```python
from build123d import *

# Parameters (mm, degrees)
F1_DEPTH = 8
F2_R     = 1.5
F3_DEPTH = 25
F5_DEPTH = 3


with BuildPart() as f1:
    # F0 (on Top) → F1 (new body)
    with BuildSketch(Plane.XY):
        with BuildLine():
            ThreePointArc((-1.3455948979, -5), (-2.7842223612, -3.1118759439), (-4.5798539423, -1.5593397432))
            ThreePointArc((-4.5798539423, -1.5593397432), (-12.5002387345, 0.4336426528), (-19.7463435047, -3.3344390538))
            ThreePointArc((-19.7463435047, -3.3344390538), (-18.6438704622, -3.0655634038), (-18, -4))
            ThreePointArc((-18, -4), (-18.2928932188, -4.7071067812), (-19, -5))
            Line((-19, -5), (-1.3455948979, -5))
        make_face()
        with BuildLine():
            ThreePointArc((-18, -4), (-18.6438704622, -3.0655634038), (-19.7463435047, -3.3344390538))
            ThreePointArc((-19.7463435047, -3.3344390538), (-19.9344365962, -3.6438704622), (-20, -4))
            ThreePointArc((-20, -4), (-19.7071067812, -4.7071067812), (-19, -5))
            ThreePointArc((-19, -5), (-18.2928932188, -4.7071067812), (-18, -4))
        make_face()
        with BuildLine():
            ThreePointArc((1.3455948979, -5), (2.7842223453, -3.1118759608), (4.5798539043, -1.5593397698))
            ThreePointArc((4.5798539043, -1.5593397698), (-2.32e-08, -3), (-4.5798539423, -1.5593397432))
            ThreePointArc((-4.5798539423, -1.5593397432), (-2.7842223612, -3.1118759439), (-1.3455948979, -5))
            Line((-1.3455948979, -5), (1.3455948979, -5))
        make_face()
        with BuildLine():
            ThreePointArc((19.7463434531, -3.3344389961), (12.5002386731, 0.43364266), (4.5798539043, -1.5593397698))
            ThreePointArc((4.5798539043, -1.5593397698), (2.7842223453, -3.1118759608), (1.3455948979, -5))
            Line((1.3455948979, -5), (19, -5))
            ThreePointArc((19, -5), (18.0874319193, -3.5910751927), (19.7463434531, -3.3344389961))
        make_face()
        with BuildLine():
            ThreePointArc((19, -5), (19.7071067812, -4.7071067812), (20, -4))
            ThreePointArc((20, -4), (19.9344365824, -3.6438704261), (19.7463434531, -3.3344389961))
            ThreePointArc((19.7463434531, -3.3344389961), (18.0874319193, -3.5910751927), (19, -5))
        make_face()
    extrude(amount=F1_DEPTH)

    # F2 (on face) → F3 (cut)
    with BuildSketch(Plane.XZ.offset(5)):
        with Locations((-15, 4)):
            Circle(F2_R)
        with Locations((15, 4)):
            Circle(F2_R)
    extrude(amount=-F3_DEPTH, mode=Mode.SUBTRACT)

    # F4 (on face) → F5 (cut)
    with BuildSketch(Plane.XZ.offset(5)):
        Polygon((-12.25, 2.4122867597), (-12.25, 5.5877132403), (-15, 7.1754264805), (-17.75, 5.5877132403), (-17.75, 2.4122867597), (-15, 0.8245735195), align=None)
        Polygon((12.25, 5.5877132403), (12.25, 2.4122867597), (15, 0.8245735195), (17.75, 2.4122867597), (17.75, 5.5877132403), (15, 7.1754264805), align=None)
    extrude(amount=-F5_DEPTH, mode=Mode.SUBTRACT)


solid = f1.part
```
Geometry: final body of the model. Coordinates: model frame, mm. A direction names the side the tool comes from. Round coordinates to 2 decimals unless told otherwise and drop trailing zeros. Loops run counter-clockwise (first coordinate to the right, second up) from the corner with the lowest first, then second, coordinate; pieces in that order, holes last.
Item 1: Section C-C, the plane z = 4. Output: boundary loops of the cut face in (x, y).
Checked values:
outline: (-19.75, -3.33) arc R1 ccw to (-19, -5) - (-17.75, -5) - (-17.75, -2) - (-16.5, -2) - (-16.5, -0.8) arc R11.5 ccw to start; (-13.5, -2) - (-12.25, -2) - (-12.25, -5) - (12.25, -5) - (12.25, -2) - (13.5, -2) - (13.5, 0.27) arc R11.5 ccw to (4.58, -1.56) arc R8 cw to (-4.58, -1.56) arc R11.5 ccw to (-13.5, 0.27) - close; (16.5, -2) - (17.75, -2) - (17.75, -5) - (19, -5) arc R1 ccw to (19.75, -3.33) arc R11.5 ccw to (16.5, -0.8) - close
Item 2: Section D-D, the plane z = 2. Output: boundary loops of the cut face in (x, y).
Checked values:
outline: (-19.75, -3.33) arc R1 ccw to (-19, -5) - (-17.04, -5) - (-17.04, -2) - (-12.96, -2) - (-12.96, -5) - (12.96, -5) - (12.96, -2) - (17.04, -2) - (17.04, -5) - (19, -5) arc R1 ccw to (19.75, -3.33) arc R11.5 ccw to (4.58, -1.56) arc R8 cw to (-4.58, -1.56) arc R11.5 ccw to start
Item 3: Section A-A, the plane y = -4.6. Output: boundary loops of the cut face in (x, z).
Checked values:
outline: (-19.8, 0) - (19.8, 0) - (19.8, 8) - (-19.8, 8) - close; hole (-17.75, 2.41) - (-15, 0.82) - (-12.25, 2.41) - (-12.25, 5.59) - (-15, 7.18) - (-17.75, 5.59) - close; hole (12.25, 2.41) - (15, 0.82) - (17.75, 2.41) - (17.75, 5.59) - (15, 7.18) - (12.25, 5.59) - close
Item 4: Contact query for flat-ended pins moving along their axis: P1, Ø1.5, axis at y = -3, z = 4.5, coming from the -X side; P2, Ø3, axis at x = 4, y = -2.5, coming from the -Z side; P3, Ø3, axis at x = 16, z = 4, coming from the -Y side; P4, Ø0.9, axis at y = -3, z = 3.5, coming from the +X side. Output: stop coordinate, or through.
Checked values:
P1: stops at x = -19.97
P2: stops at z = 0
P3: stops at y = -2
P4: stops at x = 19.84
Item 5: Line query: L1, parallel to X at y = -4.4, z = 2.75; L2, parallel to X at y = -1.05, z = 4; L3, parallel to X at y = -0.9, z = 4. Output: solid intervals per line, ascending.
Checked values:
L1: x = -19.92 to -17.75, -12.25 to 12.25, 17.75 to 19.92
L2: x = -16.95 to -16.5, -13.5 to -5.38, 5.38 to 13.5, 16.5 to 16.95
L3: x = -16.68 to -16.5, -13.5 to -5.64, 5.64 to 13.5, 16.5 to 16.68
Item 6: Reachability of faces 1 (the flat face through (16.36, -3.52, 1.61)), 2 (the cylindrical face through (12.62, 0.42, 3.94)) from +Z, -Z, +X, -X, +Y, -Y: full face, straight path, thin tool, end or side. Return the list, or none.
Checked values:
face 1: -Y
face 2: +Z, -Z, +Y
Item 7: Section B-B, the plane x = 13. Output: boundary loops of the cut face in (y, z), plus the area to 3 significant figures.
Checked values:
outline: (-5, 0) - (0.36, 0) - (0.36, 8) - (-5, 8) - (-5, 6.02) - (-2, 6.02) - (-2, 1.98) - (-5, 1.98) - close
area: 30.8 mm2
Item 8: Mould query, pull axis X, two halves, no side actions, for faces 3 (the cylindrical face through (0, -3, 4)), 4 (the flat face through (17.75, -4, 4)), 5 (the flat face through (-0.3, -3.4, 8)). Classes: released by +X, released by -X, zero draft, split by the parting line, or undercut.
Checked values:
face 3: undercut
face 4: undercut
face 5: zero draft
